Build history of the part. All positions in model axes, mm. A direction names the side the tool comes from. Give positions to 0.01 mm unless a question says otherwise; leave off trailing zeros. Order: outer loops, then holes, each group sorted by start corner. A loop starts at its lowest first (then second) coordinate and runs counter-clockwise, first axis right, second up. Notation, with made-up numbers: (19, 54) - (29, 54) arc R32 cw to (29, 85) - close; hole circle Ø4 at (-35.5, 6.25). An arc over 180 degrees is marked (long way). Answer in a Markdown table with one row per item.
```python
from build123d import *

# Parameters (mm, degrees)
SKETCH1_R           = 12.5
BOSS_EXTRUDE1_DEPTH = 7.5
SKETCH4_W           = 4
SKETCH4_H           = 27.5
BOSS_EXTRUDE3_DEPTH = 15
CIRPATTERN7_COUNT   = 6
SKETCH7_R           = 1.45
CUT_EXTRUDE2_DEPTH  = 17
CIRPATTERN9_COUNT   = 6
CUT_EXTRUDE3_REACH  = 43.398
SKETCH8_W           = 12.25
SKETCH8_H           = 12.25
SKETCH9_R           = 1.45
CUT_EXTRUDE4_DEPTH  = 10
FILLET1_R           = 1


with BuildPart() as part:
    # Sketch1 → Boss-Extrude1 (new, symmetric)
    with BuildSketch(Plane.XY):
        Circle(SKETCH1_R)
    extrude(amount=BOSS_EXTRUDE1_DEPTH, both=True)

    # Sketch4 → Boss-Extrude3 (add)
    with BuildSketch(Plane.XY.offset(7.5)):
        with Locations((-4.5, 13.75)):
            Rectangle(SKETCH4_W, SKETCH4_H)
        with Locations((4.5, 13.75)):
            Rectangle(SKETCH4_W, SKETCH4_H)
    boss_extrude3 = extrude(amount=-BOSS_EXTRUDE3_DEPTH)

    # CirPattern7: Boss-Extrude3 ×6 about axis
    cirpattern7_axis = Axis((0, 0, 0), (0, 0, 1))
    for i in range(1, CIRPATTERN7_COUNT):
        add(boss_extrude3.rotate(cirpattern7_axis, i * 360 / CIRPATTERN7_COUNT))

    # Sketch7 → Cut-Extrude2 (cut)
    with BuildSketch(Plane.ZY.offset(6.5)):
        with Locations((0, 20)):
            Circle(SKETCH7_R)
        with Locations((40, 20)):
            Circle(SKETCH7_R)
        with Locations((80, 20)):
            Circle(SKETCH7_R)
        with Locations((120, 20)):
            Circle(SKETCH7_R)
        with Locations((160, 20)):
            Circle(SKETCH7_R)
    cut_extrude2 = extrude(amount=-CUT_EXTRUDE2_DEPTH, mode=Mode.SUBTRACT)

    # CirPattern9: Cut-Extrude2 ×6 about axis
    cirpattern9_axis = Axis((0, 0, 0), (0, 0, 1))
    for i in range(1, CIRPATTERN9_COUNT):
        add(cut_extrude2.rotate(cirpattern9_axis, i * 360 / CIRPATTERN9_COUNT), mode=Mode.SUBTRACT)

    # Sketch8 → Cut-Extrude3 (cut, up to next)
    with BuildSketch(Plane.XY.offset(7.5), mode=Mode.PRIVATE) as cut_extrude3_sk1:
        Rectangle(SKETCH8_W, SKETCH8_H)
    cut_extrude3_tool1 = extrude(cut_extrude3_sk1.sketch, amount=-CUT_EXTRUDE3_REACH, mode=Mode.PRIVATE) & part.part
    add(cut_extrude3_tool1.solids().sort_by_distance((0, 0, 7.5))[0], mode=Mode.SUBTRACT)

    # Sketch9 → Cut-Extrude4 (cut)
    with BuildSketch(Plane.XY.offset(7.5)):
        with Locations((9.3125, 0)):
            Circle(SKETCH9_R)
        with Locations((0, -9.2875)):
            Circle(SKETCH9_R)
        with Locations((-9.2875, 0.025)):
            Circle(SKETCH9_R)
        with Locations((0.025, 9.3125)):
            Circle(SKETCH9_R)
    extrude(amount=-CUT_EXTRUDE4_DEPTH, mode=Mode.SUBTRACT)

    # Fillet1
    fillet1_edges = [part.edges().sort_by_distance(p)[0] for p in [
        (6.125, 6.125, 0),
        (6.125, -6.125, 0),
        (-6.125, -6.125, 0),
        (-6.125, 6.125, 0),
    ]]
    fillet(fillet1_edges, radius=FILLET1_R)


solid = part.part
```
1. Cut at C-C on z = 0. Count the separate pieces of the cut face and the enclosed holes in it, and give its area (3 significant figures).
Check result:
| item | result |
|---|---|
| separate pieces | 13 |
| enclosed holes | 5 |
| area | 939 mm² |
2. Cut at A-A on x = 4. Write the cut outline in (y, z) (3 decimals).
Check result:
| item | result |
|---|---|
| outline | (-27.5, -7.5) - (-6.125, -7.5) - (-6.125, 7.5) - (-27.5, 7.5) - close; (6.125, -7.5) - (27.5, -7.5) - (27.5, 7.5) - (6.125, 7.5) - close; hole circle Ø2.9 at (-20, 0); hole circle Ø2.9 at (20, 0) |
3. Cut at B-B on y = 17. Write the cut outline in (x, z).
Check result:
| item | result |
|---|---|
| outline | (-21.94, -7.5) - (-16.44, -7.5) - (-16.44, 7.5) - (-21.94, 7.5) - close; (-6.5, -7.5) - (-2.5, -7.5) - (-2.5, 7.5) - (-6.5, 7.5) - close; (2.5, -7.5) - (6.5, -7.5) - (6.5, 7.5) - (2.5, 7.5) - close; (16.44, -7.5) - (21.94, -7.5) - (21.94, 7.5) - (16.44, 7.5) - close |
4. Drop flat-ended pins along their axis: P1, Ø2.5, axis at x = -0.5, y = 9, coming from the +Z side; P2, Ø4, axis at y = -20, z = 0, coming from the -X side; P3, Ø2.5, axis at y = 20, z = 0, coming from the -X side; P4, Ø8, axis at x = -20.5, z = 5.5, coming from the +Y side. Give the stop position or say it passes through.
Check result:
| item | result |
|---|---|
| P1 | stops at z = 7.5 |
| P2 | stops at x = -21.36 |
| P3 | stops at x = -20.93 |
| P4 | stops at y = 19.38 |
5. Probe line 1 (Y direction, x = 0, z = 1.75) (1 decimal); line 2 (Z direction, x = -3.75, y = -20); line 3 (Y direction, x = 4.45, z = 0) (3 decimals). List the from-to ranges inside material, lowest first.
Check result:
| item | result |
|---|---|
| line 1 | y = -12.5 to -10.7, -7.8 to -6.1, 6.1 to 7.9, 10.8 to 12.5 |
| line 2 | z = -7.5 to -1.45, 1.45 to 7.5 |
| line 3 | y = -27.5 to -21.45, -18.55 to -6.125, 6.125 to 18.55, 21.45 to 27.5 |
6. Two-plate mould, pull along X, no slides. Class faces 5 (the face through (6.125, 0, 0)), 6 (the face through (-19.93, 4, 1.77)), 7 (the face through (-5, 27.5, 0)): +X half, -X half, draft (parallel to the pull), parting line (faces both ways), or undercut.
Check result:
| item | result |
|---|---|
| face 5 | undercut |
| face 6 | -X half |
| face 7 | draft |
7. Which spindle directions (+Z, -Z, +X, -X, +Y, -Y) get a long thin tool onto all of the face, cutting with end or side? Do faces 1 (the face through (-6.5, 19, 2)), 2 (the face through (0, -9, -2.5)), 3 (the face through (13.43, -15.26, 1.77)), 4 (the face through (15.87, -12.05, 1.77)). Say none if no direction does.
Check result:
| item | result |
|---|---|
| face 1 | +Z, -Z, +Y |
| face 2 | +Z |
| face 3 | +Z, -Z, -Y |
| face 4 | +Z, -Z |
